Could you check a few things on this model? Use its own coordinates, in mm. A direction names the side the tool comes from. Give positions to 0.01 mm unless a question says otherwise; leave off trailing zeros. Loops run counter-clockwise (first coordinate to the right, second up) from the corner with the lowest first, then second, coordinate; pieces in that order, holes last. Notation, with made-up numbers: (-5, 83) - (39, 83) arc R16 cw to (39, 92) - close; hole circle Ø8 at (-30, -17). An arc over 180 degrees is marked (long way). Use CSV: the item, a comma, the result in double quotes.
from build123d import *

# Parameters (mm, degrees)
BOSS_EXTRUDE1_DEPTH = 2.5
CUT_EXTRUDE1_REACH  = 111.75
SKETCH2_R           = 4.25


with BuildPart() as part:
    # Sketch1 → Boss-Extrude1 (new, symmetric)
    with BuildSketch(Plane(origin=(0, 0, 0), x_dir=(0, 1, 0), z_dir=(0, 0, 1))):
        Polygon((25.5, 50), (-25.5, 50), (-25.5, 40), (-20.5, 40), (-20.5, 30), (-25.5, 30), (-25.5, 20), (-28, -25), (-28, -40), (-23, -40), (-23, -50), (-28, -50), (-28, -81), (-23, -81), (-23, -91), (-28, -91), (-28, -106), (28, -106), (28, -91), (23, -91), (23, -81), (28, -81), (28, -50), (23, -50), (23, -40), (28, -40), (28, -25), (25.5, 20), (25.5, 30), (20.5, 30), (20.5, 40), (25.5, 40), align=None)
    extrude(amount=BOSS_EXTRUDE1_DEPTH, both=True)

    # Sketch2 → Cut-Extrude1 (cut, up to next)
    with BuildSketch(Plane.XY.offset(2.5), mode=Mode.PRIVATE) as cut_extrude1_sk1:
        with Locations((-35, 0)):
            Circle(SKETCH2_R)
    cut_extrude1_tool1 = extrude(cut_extrude1_sk1.sketch, amount=-CUT_EXTRUDE1_REACH, mode=Mode.PRIVATE) & part.part
    # Sketch2 → Cut-Extrude1 (cut, up to next)
    with BuildSketch(Plane.XY.offset(2.5), mode=Mode.PRIVATE) as cut_extrude1_sk2:
        with Locations((45, 0)):
            Circle(SKETCH2_R)
    cut_extrude1_tool2 = extrude(cut_extrude1_sk2.sketch, amount=-CUT_EXTRUDE1_REACH, mode=Mode.PRIVATE) & part.part
    # Sketch2 → Cut-Extrude1 (cut, up to next)
    with BuildSketch(Plane.XY.offset(2.5), mode=Mode.PRIVATE) as cut_extrude1_sk3:
        with Locations((85, 0)):
            Circle(SKETCH2_R)
    cut_extrude1_tool3 = extrude(cut_extrude1_sk3.sketch, amount=-CUT_EXTRUDE1_REACH, mode=Mode.PRIVATE) & part.part
    # Sketch2 → Cut-Extrude1 (cut, up to next)
    with BuildSketch(Plane.XY.offset(2.5), mode=Mode.PRIVATE) as cut_extrude1_sk4:
        with Locations((90, 0)):
            Circle(SKETCH2_R)
    cut_extrude1_tool4 = extrude(cut_extrude1_sk4.sketch, amount=-CUT_EXTRUDE1_REACH, mode=Mode.PRIVATE) & part.part
    # Sketch2 → Cut-Extrude1 (cut, up to next)
    with BuildSketch(Plane.XY.offset(2.5), mode=Mode.PRIVATE) as cut_extrude1_sk5:
        with Locations((50, 0)):
            Circle(SKETCH2_R)
    cut_extrude1_tool5 = extrude(cut_extrude1_sk5.sketch, amount=-CUT_EXTRUDE1_REACH, mode=Mode.PRIVATE) & part.part
    # Sketch2 → Cut-Extrude1 (cut, up to next)
    with BuildSketch(Plane.XY.offset(2.5), mode=Mode.PRIVATE) as cut_extrude1_sk6:
        with Locations((-30, 0)):
            Circle(SKETCH2_R)
    cut_extrude1_tool6 = extrude(cut_extrude1_sk6.sketch, amount=-CUT_EXTRUDE1_REACH, mode=Mode.PRIVATE) & part.part
    # Sketch2 → Cut-Extrude1 (cut, up to next)
    with BuildSketch(Plane.XY.offset(2.5), mode=Mode.PRIVATE) as cut_extrude1_sk7:
        with Locations((80, 0)):
            Circle(SKETCH2_R)
    cut_extrude1_tool7 = extrude(cut_extrude1_sk7.sketch, amount=-CUT_EXTRUDE1_REACH, mode=Mode.PRIVATE) & part.part
    # Sketch2 → Cut-Extrude1 (cut, up to next)
    with BuildSketch(Plane.XY.offset(2.5), mode=Mode.PRIVATE) as cut_extrude1_sk8:
        with Locations((40, 0)):
            Circle(SKETCH2_R)
    cut_extrude1_tool8 = extrude(cut_extrude1_sk8.sketch, amount=-CUT_EXTRUDE1_REACH, mode=Mode.PRIVATE) & part.part
    # Sketch2 → Cut-Extrude1 (cut, up to next)
    with BuildSketch(Plane.XY.offset(2.5), mode=Mode.PRIVATE) as cut_extrude1_sk9:
        with Locations((-40, 0)):
            Circle(SKETCH2_R)
    cut_extrude1_tool9 = extrude(cut_extrude1_sk9.sketch, amount=-CUT_EXTRUDE1_REACH, mode=Mode.PRIVATE) & part.part
    add(cut_extrude1_tool1.solids().sort_by_distance((-35, 0, 2.5))[0], mode=Mode.SUBTRACT)
    add(cut_extrude1_tool2.solids().sort_by_distance((45, 0, 2.5))[0], mode=Mode.SUBTRACT)
    add(cut_extrude1_tool3.solids().sort_by_distance((85, 0, 2.5))[0], mode=Mode.SUBTRACT)
    add(cut_extrude1_tool4.solids().sort_by_distance((90, 0, 2.5))[0], mode=Mode.SUBTRACT)
    add(cut_extrude1_tool5.solids().sort_by_distance((50, 0, 2.5))[0], mode=Mode.SUBTRACT)
    add(cut_extrude1_tool6.solids().sort_by_distance((-30, 0, 2.5))[0], mode=Mode.SUBTRACT)
    add(cut_extrude1_tool7.solids().sort_by_distance((80, 0, 2.5))[0], mode=Mode.SUBTRACT)
    add(cut_extrude1_tool8.solids().sort_by_distance((40, 0, 2.5))[0], mode=Mode.SUBTRACT)
    add(cut_extrude1_tool9.solids().sort_by_distance((-40, 0, 2.5))[0], mode=Mode.SUBTRACT)


solid = part.part
1) Suppose I cut it at B-B (x = -28). Please give me the cut outline in (y, z).
Answer below:
outline,"(-25.5, -2.5) - (-3.75, -2.5) - (-3.75, 2.5) - (-25.5, 2.5) - close; (3.75, -2.5) - (25.5, -2.5) - (25.5, 2.5) - (3.75, 2.5) - close"
2) We'd pull the mould along Y, two halves only. Please class faces 1 (the cylindrical face through (-35.04, -4.25, 0.04)), 2 (the flat face through (98, -28, 0)), 3 (the flat face through (-30, -23, 0)): +Y half, -Y half, draft (parallel to the pull), parting line (faces both ways), or undercut.
Answer below:
face 1,"undercut"
face 2,"-Y half"
face 3,"draft"
3) Suppose I cut it at C-C (z = -0.4). State how many separate pieces and enclosed holes the cut face has, plus the area to 3 significant figures.
Answer below:
separate pieces,"1"
enclosed holes,"3"
area,"7,760 mm2"
4) Which directions (+Z, -Z, +X, -X, +Y, -Y) give clear straight access to the entire face, cutting with the end or side of a thin tool? Please do faces 4 (the flat face through (-40, -23, 0)), 5 (the flat face through (45, 23, 0)), 6 (the flat face through (-45, 25.5, 0)), 7 (the cylindrical face through (45.04, 4.25, 0.04)).
Answer below:
face 4,"+Z, -Z, -Y"
face 5,"+Z, -Z, +Y"
face 6,"+Z, -Z, -X, +Y"
face 7,"+Z, -Z"
5) Suppose I cut it at D-D (x = 84.5). Please give me the cut outline in (y, z).
Answer below:
outline,"(-23, -2.5) - (-4.22, -2.5) - (-4.22, 2.5) - (-23, 2.5) - close; (4.22, -2.5) - (23, -2.5) - (23, 2.5) - (4.22, 2.5) - close"
6) Suppose I cut it at A-A (y = 0). Please give me the cut outline in (x, z), plus the area to 4 significant figures.
Answer below:
outline,"(-50, -2.5) - (-44.25, -2.5) - (-44.25, 2.5) - (-50, 2.5) - close; (-25.75, -2.5) - (35.75, -2.5) - (35.75, 2.5) - (-25.75, 2.5) - close; (54.25, -2.5) - (75.75, -2.5) - (75.75, 2.5) - (54.25, 2.5) - close; (94.25, -2.5) - (106, -2.5) - (106, 2.5) - (94.25, 2.5) - close"
area,"502.5 mm2"
7) I'm going to push flat-ended pins straight in: P1, Ø2.5, axis at y = 26, z = 0.5, coming from the -X side; P2, Ø2, axis at x = -3.5, z = -0.5, coming from the +Y side. Where does each tip first touch, or does it pass through?
Answer below:
P1,"stops at x = -50"
P2,"stops at y = 26.47"
8) I need wall thicknesses on line 1 along X through (y, z) = (0, -1); line 2 along X through (y, z) = (25, 1.3); line 3 along X through (y, z) = (-22, 2.3). Which ranges of each line are inside material? Lowest first, please.
Answer below:
line 1,"x = -50 to -44.25, -25.75 to 35.75, 54.25 to 75.75, 94.25 to 106"
line 2,"x = -50 to -40, -30 to 40, 50 to 81, 91 to 106"
line 3,"x = -50 to -40, -30 to 106"
